Autodesk Inventor part; units mm, degrees
ref_plane "YZ Plane" through (0, 0, 0) normal (1, 0, 0) x (0, 1, 0)
ref_plane "XZ Plane" through (0, 0, 0) normal (0, 1, 0) x (-1, 0, 0)
ref_plane "XY Plane" through (0, 0, 0) normal (0, 0, 1) x (1, 0, 0)
sketch "草圖1" plane through (0, 0, 0) normal (0, 0, 1) x (1, 0, 0)
  circle A0 centre (0, 0) radius 135
  circle A1 centre (0, 0) radius 153.85
  dimension "d0" = 270
  dimension "d1" = 18.85
  dimension "d2" = 307.7
extrude "擠出1" add sketch "草圖1" along normal blind 3
chamfer "倒角1" distance 0.3 angle 45 2 edges at (-135, 0, 3) (-135, 0, 0)
chamfer "倒角2" distance 0.5 angle 45 2 edges at (-153.85, 0, 3) (-153.85, 0, 0)
properties part number "鐵弗龍間隔環"
CAD build for the part. Positions are in the model's coordinates, mm. Round coordinates to 2 decimals unless told otherwise and drop trailing zeros. Order: outer loops, then holes, each group sorted by start corner. A loop starts at its lowest first (then second) coordinate and runs counter-clockwise, first axis right, second up.
Q1. Slice it at C-C (z = 1.45). Write the cut outline in (x, y).
Q2. Two-plate mould, pull along Y, no slides. Class faces 1 (the flat face through (-1, -136, 3)), 2 (the cylindrical face through (-33.35, 150.19, 1.49)), 3 (the cylindrical face through (-107.13, 82.15, 1.48)): pulls with the +Y half, pulls with the -Y half, needs draft (parallel to the pull), parting line crosses it, or undercut.
Q3. Drop a flat-ended pin along its axis: pin 1 (4 mm diameter, centred on x = -109.5, y = 100, fed in from -Z). Give the stop position or say it passes through.
Q4. Wall check: L1, parallel to Y at x = 0, z = 1.3; L2, parallel to X at y = -98, z = 0.4; L3, parallel to Y at x = -107, z = 0.3. Give the ranges that are in metal, low to high.
Q5. Slice it at A-A (y = 0). Write the cut outline in (x, z).
Results below:
1. outline: circle Ø307.7 at (0, 0); hole circle Ø270 at (0, 0)
2. face 1: needs draft
2. face 2: parting line crosses it
2. face 3: undercut
3. pin 1: stops at z = 0
4. L1: y = -153.85 to -135, 135 to 153.85
4. L2: x = -118.47 to -92.85, 92.85 to 118.47
4. L3: y = -110.27 to -82.32, 82.32 to 110.27
5. outline: (-153.85, 0.5) - (-153.35, 0) - (-135.3, 0) - (-135, 0.3) - (-135, 2.7) - (-135.3, 3) - (-153.35, 3) - (-153.85, 2.5) - close; (135, 0.3) - (135.3, 0) - (153.35, 0) - (153.85, 0.5) - (153.85, 2.5) - (153.35, 3) - (135.3, 3) - (135, 2.7) - close
